Verification items for the finished model (mm, model axes). A direction names the side the tool comes from. Give positions to 0.01 mm unless a question says otherwise; leave off trailing zeros. Order: outer loops, then holes, each group sorted by start corner. A loop starts at its lowest first (then second) coordinate and runs counter-clockwise, first axis right, second up. Notation, with made-up numbers: M 20,77.25 L 32,77.25 A20 cw 32,114.25 Z; hole C 43.5,87 d6. An arc over 180 degrees is marked long. Answer as a JSON object with one key per item and string values.
```python
from build123d import *

# Parameters (mm, degrees)
BASE_FLANGE1_DEPTH      = 25.273
CUT_EXTRUDE1_DEPTH      = 117.714472655
CUT_EXTRUDE1_DEPTH_BACK = 117.714472655
SKETCH6_W               = 13.208
SKETCH6_H               = 3.048
CUT_EXTRUDE2_DEPTH      = 182.766885422
CUT_EXTRUDE2_DEPTH_BACK = 182.766885422
SKETCH7_W               = 3.048
SKETCH7_H               = 13.208
FILLET1_R               = 2.54
SKETCH8_R               = 0.7747
CUT_EXTRUDE3_DEPTH      = 182.766885422
CUT_EXTRUDE5_REACH      = 186.487
SKETCH10_R              = 1.651


# Sheet-metal steps are written as plain solids
with BuildPart() as part:
    # Sketch1 → Base-Flange1 (new, symmetric)
    with BuildSketch(Plane.XY):
        with BuildLine():
            Line((79.441088515, 78.607212609), (79.441088515, 2.667))
            ThreePointArc((79.441088515, 2.667), (78.6599423, 0.781146215), (76.774088515, 0))
            Line((76.774088515, 0), (-76.774088515, 0))
            ThreePointArc((-76.774088515, 0), (-78.6599423, 0.781146215), (-79.441088515, 2.667))
            Line((-79.441088515, 2.667), (-79.441088515, 78.607212609))
            Line((-79.441088515, 78.607212609), (-82.489088515, 78.607212609))
            Line((-82.489088515, 78.607212609), (-82.489088515, 2.667))
            ThreePointArc((-82.489088515, 2.667), (-80.815203769, -1.374115254), (-76.774088515, -3.048))
            Line((-76.774088515, -3.048), (76.774088515, -3.048))
            ThreePointArc((76.774088515, -3.048), (80.815203769, -1.374115254), (82.489088515, 2.667))
            Line((82.489088515, 2.667), (82.489088515, 78.607212609))
            Line((82.489088515, 78.607212609), (79.441088515, 78.607212609))
        make_face()
    extrude(amount=BASE_FLANGE1_DEPTH, both=True)

    # Sketch6 → Cut-Extrude1 (cut, two sides: drawn at the far end of the back side and taken through both)
    with BuildSketch(Plane(origin=(0, 0, 0), x_dir=(1, 0, 0), z_dir=(0, 1, 0)).offset(-CUT_EXTRUDE1_DEPTH_BACK)):
        with Locations((-57.404, 23.749)):
            Rectangle(SKETCH6_W, SKETCH6_H)
        with Locations((-57.404, -23.749)):
            Rectangle(SKETCH6_W, SKETCH6_H)
        with Locations((57.404, -23.749)):
            Rectangle(SKETCH6_W, SKETCH6_H)
        with Locations((57.404, 23.749)):
            Rectangle(SKETCH6_W, SKETCH6_H)
    extrude(amount=CUT_EXTRUDE1_DEPTH + CUT_EXTRUDE1_DEPTH_BACK, mode=Mode.SUBTRACT)

    # Sketch7 → Cut-Extrude2 (cut, two sides: drawn at the far end of the back side and taken through both)
    with BuildSketch(Plane(origin=(-79.441088515, 0, 0), x_dir=(0, 0, -1), z_dir=(1, 0, 0)).offset(-CUT_EXTRUDE2_DEPTH_BACK)):
        with Locations((-23.749, 28.956)):
            Rectangle(SKETCH7_W, SKETCH7_H)
        with Locations((23.749, 28.956)):
            Rectangle(SKETCH7_W, SKETCH7_H)
    extrude(amount=CUT_EXTRUDE2_DEPTH + CUT_EXTRUDE2_DEPTH_BACK, mode=Mode.SUBTRACT)

    # Fillet1
    fillet1_edges = [part.edges().sort_by_distance(p)[0] for p in [
        (80.965088515, 78.607212609, -25.273),
        (-80.965088515, 78.607212609, -25.273),
        (80.965088515, 78.607212609, 25.273),
        (-80.965088515, 78.607212609, 25.273),
    ]]
    fillet(fillet1_edges, radius=FILLET1_R)

    # Sketch8 → Cut-Extrude3 (cut, through all)
    with BuildSketch(Plane.ZY.offset(-79.441088515)):
        with Locations(Location((0, 58.625617182, 0), (0, 0, 270))):
            Circle(SKETCH8_R)
        with Locations(Location((0, 71.325617182, 0), (0, 0, 270))):
            Circle(SKETCH8_R)
    extrude(amount=-CUT_EXTRUDE3_DEPTH, mode=Mode.SUBTRACT)

    # Sketch10 → Cut-Extrude5 (cut, up to next)
    with BuildSketch(Plane.ZY.offset(82.489088515), mode=Mode.PRIVATE) as cut_extrude5_sk1:
        with Locations(Location((11.90625, 68.447212609, 0), (0, 0, 270))):
            Circle(SKETCH10_R)
    cut_extrude5_tool1 = extrude(cut_extrude5_sk1.sketch, amount=-CUT_EXTRUDE5_REACH, mode=Mode.PRIVATE) & part.part
    # Sketch10 → Cut-Extrude5 (cut, up to next)
    with BuildSketch(Plane.ZY.offset(82.489088515), mode=Mode.PRIVATE) as cut_extrude5_sk2:
        with Locations(Location((-11.90625, 68.447212609, 0), (0, 0, 270))):
            Circle(SKETCH10_R)
    cut_extrude5_tool2 = extrude(cut_extrude5_sk2.sketch, amount=-CUT_EXTRUDE5_REACH, mode=Mode.PRIVATE) & part.part
    add(cut_extrude5_tool1.solids().sort_by_distance((-82.489089, 68.447213, 11.90625))[0], mode=Mode.SUBTRACT)
    add(cut_extrude5_tool2.solids().sort_by_distance((-82.489089, 68.447213, -11.90625))[0], mode=Mode.SUBTRACT)


solid = part.part
```
Q1. Gauge pin test, flat ends, axial feed: pin 1 Ø2.5 at (y, z) = (-1, -23) entering from -X; pin 2 Ø3.5 at (x, z) = (-81, 23) entering from -Y; pin 3 Ø1.5 at (y, z) = (-1, -23) entering from -X. Record the tip position at first contact, or that the pin passes through.
Resolved:
{"pin 1": "stops at x = -81.95", "pin 2": "stops at y = -2.48", "pin 3": "stops at x = -81.69"}
Q2. Section check D-D on x = -56.5. Record the cut outline in (y, z) (3 decimals), then the cut area to 3 significant figures.
Resolved:
{"outline": "M -3.048,-22.225 L 0,-22.225 L 0,22.225 L -3.048,22.225 Z", "area": "135 mm²"}
Q3. Section check A-A on y = 12. Record the cut outline in (x, z), then the cut area to 3 significant figures.
Resolved:
{"outline": "M -82.49,-25.27 L -79.44,-25.27 L -79.44,25.27 L -82.49,25.27 Z; M 79.44,-25.27 L 82.49,-25.27 L 82.49,25.27 L 79.44,25.27 Z", "area": "308 mm²"}
Q4. Material ranges on L1, parallel to X at y = 43, z = 9; L2, parallel to Y at x = -22.5, z = 10, recorded low to high.
Resolved:
{"L1": "x = -82.49 to -79.44, 79.44 to 82.49", "L2": "y = -3.05 to 0"}
Q5. Section check B-B on z = 4. Record the cut outline in (x, y) (3 decimals), then the cut area to 3 significant figures.
Resolved:
{"outline": "M -82.489,2.667 A5.715 ccw -76.774,-3.048 L 76.774,-3.048 A5.715 ccw 82.489,2.667 L 82.489,78.607 L 79.441,78.607 L 79.441,2.667 A2.667 cw 76.774,0 L -76.774,0 A2.667 cw -79.441,2.667 L -79.441,78.607 L -82.489,78.607 Z", "area": "971 mm²"}
Q6. Section check C-C on x = -7. Record the cut outline in (y, z), then the cut area to 3 significant figures.
Resolved:
{"outline": "M -3.05,-25.27 L 0,-25.27 L 0,25.27 L -3.05,25.27 Z", "area": "154 mm²"}
Q7. Release check for a two-part mould opening along X. For faces 6 (the face through (82.489, 40, 0)), 7 (the face through (-81, 22.352, 24)), 8 (the face through (79.441, 41, 0)), 9 (the face through (50.8, -2, 24)) record: +X half, -X half, draft (parallel to the pull), parting line (faces both ways), or undercut.
Resolved:
{"face 6": "+X half", "face 7": "draft", "face 8": "undercut", "face 9": "undercut"}
Q8. Tool access check on faces 1 (the face through (81, 56, 25.273)), 2 (the face through (64.008, -2, 24)), 3 (the face through (-57, -2, -22.225)), 4 (the face through (81, 22.352, 24)), 5 (the face through (-81, 35.56, -24)). Record the directions out of +Z, -Z, +X, -X, +Y, -Y that give a thin tool (end or side, any length) a straight path to the whole face; none if there is none.
Resolved:
{"face 1": "+Z, +X, -X, +Y, -Y", "face 2": "+Z, +Y, -Y", "face 3": "-Z, +Y, -Y", "face 4": "+Z, +X, -X", "face 5": "-Z, +X, -X"}
